```python
from build123d import *

# Parameters (mm, degrees)
SKETCH_1_W                = 73.9
SKETCH_1_H                = 56.9
EXTRUDE_1_DEPTH           = 4
HOLE_WIZARD_1_D           = 3
HOLE_WIZARD_1_CBORE_D     = 6
HOLE_WIZARD_1_CBORE_DEPTH = 2.2
SKETCH_4_W                = 7
SKETCH_4_H                = 25.95
SKETCH_4_W_2              = 33.45
SKETCH_4_H_2              = 7
SKETCH_4_H_3              = 23.95
EXTRUDE_2_DEPTH           = 2
HOLE_WIZARD_2_D           = 3.2
CHAMFER_1_SIZE            = 1
CHAMFER_1_SIZE_2          = 2
CHAMFER_2_SIZE            = 2
CHAMFER_2_SIZE_2          = 1
CHAMFER_3_SIZE            = 2
CHAMFER_3_SIZE_2          = 1
SKETCH_7_W                = 2
SKETCH_7_H                = 1
SKETCH_7_W_2              = 1
SKETCH_7_H_2              = 2
EXTRUDE_3_DEPTH           = 2
FILLET_3_R                = 1
FILLET_4_R                = 1


with BuildPart() as part:
    # 草图1 → 凸台-拉伸1 (new body)
    with BuildSketch(Plane.XY):
        Rectangle(SKETCH_1_W, SKETCH_1_H)
    extrude(amount=EXTRUDE_1_DEPTH)

    # 孔1 (through all)
    with Locations(Plane(origin=(-10, 9.25, 4), x_dir=(1, 0, 0), z_dir=(0, 0, 1))):
        with Locations((0, 0), (20, 0), (20, -18.5), (0, -18.5)):
            CounterBoreHole(HOLE_WIZARD_1_D / 2, HOLE_WIZARD_1_CBORE_D / 2, HOLE_WIZARD_1_CBORE_DEPTH)

    # 草图4 → 凸台-拉伸2 (add)
    with BuildSketch(Plane(origin=(0, 0, 0), x_dir=(-1, 0, 0), z_dir=(0, 0, -1))):
        with BuildLine():
            Line((3.5, 28.45), (3.5, 35.5))
            ThreePointArc((3.5, 35.5), (0, 39), (-3.5, 35.5))
            Line((-3.5, 35.5), (-3.5, 28.45))
            Line((-3.5, 28.45), (3.5, 28.45))
        make_face()
        with Locations((0, 15.475)):
            Rectangle(SKETCH_4_W, SKETCH_4_H)
        with Locations((20.225, -1)):
            Rectangle(SKETCH_4_W_2, SKETCH_4_H_2)
        with BuildLine():
            Line((43, 2.5), (36.95, 2.5))
            Line((36.95, 2.5), (36.95, -4.5))
            Line((36.95, -4.5), (43, -4.5))
            ThreePointArc((43, -4.5), (46.5, -1), (43, 2.5))
        make_face()
        with Locations((0, -1)):
            Rectangle(SKETCH_4_W, SKETCH_4_H_2)
        with Locations((-20.225, -1)):
            Rectangle(SKETCH_4_W_2, SKETCH_4_H_2)
        with Locations((0, -16.475)):
            Rectangle(SKETCH_4_W, SKETCH_4_H_3)
        with BuildLine():
            Line((-36.95, -4.5), (-36.95, 2.5))
            Line((-36.95, 2.5), (-43, 2.5))
            ThreePointArc((-43, 2.5), (-46.5, -1), (-43, -4.5))
            Line((-43, -4.5), (-36.95, -4.5))
        make_face()
        with BuildLine():
            Line((3.5, -35.5), (3.5, -28.45))
            Line((3.5, -28.45), (-3.5, -28.45))
            Line((-3.5, -28.45), (-3.5, -35.5))
            ThreePointArc((-3.5, -35.5), (0, -39), (3.5, -35.5))
        make_face()
    extrude(amount=EXTRUDE_2_DEPTH)

    # 孔2 (through all)
    with Locations(Plane(origin=(43, -1, -2), x_dir=(-1, 0, 0), z_dir=(0, 0, -1))):
        with Locations((0, 0), (43, 36.5), (86, 0), (43, -34.5)):
            Hole(HOLE_WIZARD_2_D / 2)

    # 倒角1
    # the kernel refuses this chamfer: 2, 1 mm, written as the material it adds along each edge
    with BuildSketch(Plane(origin=(-3.5, -2.679657748, 0), x_dir=(-0.9976223042390326, 0, 0.06891834360170879), z_dir=(0, 1, 0))) as chamfer_1_piece_1:
        Polygon((CHAMFER_1_SIZE * 0.997622304239, -CHAMFER_1_SIZE * 0.0689183436017), (-CHAMFER_1_SIZE_2 * 0.0689183436017, -CHAMFER_1_SIZE_2 * 0.997622304239), (0, 0), align=None)
    extrude(amount=31.129657748)
    with BuildSketch(Plane(origin=(-36.95, 2.5, 0), x_dir=(0, 0.9976223042390326, 0.06891834360170879), z_dir=(1, 0, 0))) as chamfer_1_piece_2:
        Polygon((CHAMFER_1_SIZE * 0.997622304239, -CHAMFER_1_SIZE * 0.0689183436017), (-CHAMFER_1_SIZE_2 * 0.0689183436017, -CHAMFER_1_SIZE_2 * 0.997622304239), (0, 0), align=None)
    extrude(amount=38.629657748)

    # 倒角2
    # the kernel refuses this chamfer: 2, 1 mm, written as the material it adds along each edge
    with BuildSketch(Plane(origin=(-3.5, 0.679657748, 0), x_dir=(0.017268075123668084, 0, -0.9998508956747119), z_dir=(0, -1, 0))) as chamfer_2_piece_1:
        Polygon((CHAMFER_2_SIZE * 0.999850895675, -CHAMFER_2_SIZE * 0.0172680751237), (-CHAMFER_2_SIZE_2 * 0.0172680751237, -CHAMFER_2_SIZE_2 * 0.999850895675), (0, 0), align=None)
    extrude(amount=29.129657748)
    with BuildSketch(Plane(origin=(-36.95, -4.5, 0), x_dir=(0, 0.017268075123667872, -0.9998508956747119), z_dir=(1, 0, 0))) as chamfer_2_piece_2:
        Polygon((CHAMFER_2_SIZE * 0.999850895675, -CHAMFER_2_SIZE * 0.0172680751237), (-CHAMFER_2_SIZE_2 * 0.0172680751237, -CHAMFER_2_SIZE_2 * 0.999850895675), (0, 0), align=None)
    extrude(amount=38.629657748)

    # 倒角3
    # the kernel refuses this chamfer: 2, 1 mm, written as the material it adds along each edge
    with BuildSketch(Plane(origin=(3.5, -28.45, 0), x_dir=(-0.0172680751236683, 0, -0.9998508956747119), z_dir=(0, 1, 0))) as chamfer_3_piece_1:
        Polygon((CHAMFER_3_SIZE * 0.999850895675, -CHAMFER_3_SIZE * 0.0172680751237), (-CHAMFER_3_SIZE_2 * 0.0172680751237, -CHAMFER_3_SIZE_2 * 0.999850895675), (0, 0), align=None)
    extrude(amount=29.129657748)
    with BuildSketch(Plane(origin=(-1.679657748, -4.5, 0), x_dir=(0, 0.0172680751236683, -0.9998508956747119), z_dir=(1, 0, 0)), Plane(origin=(36.95, 2.5, 0), x_dir=(0, -0.017268075123667872, -0.9998508956747119), z_dir=(-1, 0, 0))) as chamfer_3_piece_2:
        Polygon((CHAMFER_3_SIZE * 0.999850895675, -CHAMFER_3_SIZE * 0.0172680751237), (-CHAMFER_3_SIZE_2 * 0.0172680751237, -CHAMFER_3_SIZE_2 * 0.999850895675), (0, 0), align=None)
    extrude(amount=38.629657748)
    with BuildSketch(Plane(origin=(3.5, -2.679657748, 0), x_dir=(-0.017268075123668084, 0, -0.9998508956747119), z_dir=(0, 1, 0))) as chamfer_3_piece_3:
        Polygon((CHAMFER_3_SIZE * 0.999850895675, -CHAMFER_3_SIZE * 0.0172680751237), (-CHAMFER_3_SIZE_2 * 0.0172680751237, -CHAMFER_3_SIZE_2 * 0.999850895675), (0, 0), align=None)
    extrude(amount=31.129657748)

    # 草图7 → 凸台-拉伸3 (add)
    # profile 1 of 6: a face of its own
    with BuildSketch(Plane(origin=(0, 0, 0), x_dir=(-1, 0, 0), z_dir=(0, 0, -1))):
        with BuildLine():
            Line((-36.95, 4.5), (-43, 4.5))
            ThreePointArc((-43, 4.5), (-48.5, -1), (-43, -6.5))
            Line((-43, -6.5), (-34.95, -6.5))
            Line((-34.95, -6.5), (-34.95, 3.5))
            Line((-34.95, 3.5), (-36.95, 3.5))
            Line((-36.95, 3.5), (-36.95, 4.5))
        make_face()
        with BuildLine():
            Line((-43, 2.5), (-36.95, 2.5))
            Line((-36.95, 2.5), (-36.95, -4.5))
            Line((-36.95, -4.5), (-43, -4.5))
            ThreePointArc((-43, -4.5), (-46.5, -1), (-43, 2.5))
        make_face(mode=Mode.SUBTRACT)
    # profile 2 of 6: a face of its own
    with BuildSketch(Plane(origin=(0, 0, 0), x_dir=(-1, 0, 0), z_dir=(0, 0, -1))):
        with Locations((-35.95, 4)):
            Rectangle(SKETCH_7_W, SKETCH_7_H)
    # profile 3 of 6: a face of its own
    with BuildSketch(Plane(origin=(0, 0, 0), x_dir=(-1, 0, 0), z_dir=(0, 0, -1))):
        with BuildLine():
            Line((-5.5, -35.5), (-5.5, -26.45))
            Line((-5.5, -26.45), (5.5, -26.45))
            Line((5.5, -26.45), (5.5, -35.5))
            ThreePointArc((5.5, -35.5), (0, -41), (-5.5, -35.5))
        make_face()
        with BuildLine():
            ThreePointArc((-3.5, -35.5), (0, -39), (3.5, -35.5))
            Line((3.5, -35.5), (3.5, -28.45))
            Line((3.5, -28.45), (-3.5, -28.45))
            Line((-3.5, -28.45), (-3.5, -35.5))
        make_face(mode=Mode.SUBTRACT)
    # profile 4 of 6: a face of its own
    with BuildSketch(Plane(origin=(0, 0, 0), x_dir=(-1, 0, 0), z_dir=(0, 0, -1))):
        with BuildLine():
            Line((43, -6.5), (34.95, -6.5))
            Line((34.95, -6.5), (34.95, 4.5))
            Line((34.95, 4.5), (43, 4.5))
            ThreePointArc((43, 4.5), (48.5, -1), (43, -6.5))
        make_face()
        with BuildLine():
            ThreePointArc((43, -4.5), (46.5, -1), (43, 2.5))
            Line((43, 2.5), (36.95, 2.5))
            Line((36.95, 2.5), (36.95, -4.5))
            Line((36.95, -4.5), (43, -4.5))
        make_face(mode=Mode.SUBTRACT)
    # profile 5 of 6: a face of its own
    with BuildSketch(Plane(origin=(0, 0, 0), x_dir=(-1, 0, 0), z_dir=(0, 0, -1))):
        with BuildLine():
            Line((-5.5, 35.5), (-5.5, 28.45))
            Line((-5.5, 28.45), (-4.5, 28.45))
            Line((-4.5, 28.45), (-4.5, 26.45))
            Line((-4.5, 26.45), (5.5, 26.45))
            Line((5.5, 26.45), (5.5, 35.5))
            ThreePointArc((5.5, 35.5), (0, 41), (-5.5, 35.5))
        make_face()
        with BuildLine():
            Line((3.5, 35.5), (3.5, 28.45))
            Line((3.5, 28.45), (-3.5, 28.45))
            Line((-3.5, 28.45), (-3.5, 35.5))
            ThreePointArc((-3.5, 35.5), (0, 39), (3.5, 35.5))
        make_face(mode=Mode.SUBTRACT)
    # profile 6 of 6: a face of its own
    with BuildSketch(Plane(origin=(0, 0, 0), x_dir=(-1, 0, 0), z_dir=(0, 0, -1))):
        with Locations((-5, 27.45)):
            Rectangle(SKETCH_7_W_2, SKETCH_7_H_2)
    extrude(amount=EXTRUDE_3_DEPTH)

    # 圆角3
    fillet_3_edges = [part.edges().sort_by_distance(p)[0] for p in [
        (-34.95, -6.5, -1),
        (-34.95, 4.5, -1),
        (5.5, -26.45, -1),
        (-5.5, -26.45, -1),
        (-5.5, 26.45, -1),
        (5.5, 26.45, -1),
        (34.95, 4.5, -1),
        (34.95, -6.5, -1),
    ]]
    fillet(fillet_3_edges, radius=FILLET_3_R)

    # 圆角4
    fillet_4_edges = [part.edges().sort_by_distance(p)[0] for p in [
        (36.95, -28.45, 2),
        (-36.95, -28.45, 2),
        (-36.95, 28.45, 2),
        (36.95, 28.45, 2),
    ]]
    fillet(fillet_4_edges, radius=FILLET_4_R)


solid = part.part
```
Check sheet for the modelled part. Datum: model origin and axes. Units: mm. A direction names the side the tool comes from. Coordinates: 2 decimals unless noted, no trailing zeros. Order: outer loops, then holes, each group sorted by start corner. A loop starts at its lowest first (then second) coordinate and runs counter-clockwise, first axis right, second up. Notation, with made-up numbers: (64, 47) -> (104, 47) arc R8 cw to (104, 51) -> close; hole circle Ø6 at (26.5, 41). An arc over 180 degrees is marked (long way). Write item = value, one per line. Start each with the question number.
1) Access from +Z, -Z, +X, -X, +Y, -Y to the whole of each face (thin tool, end or side, straight path). Record for faces 1 (the flat face through (-1, 0, 4)), 2 (the flat face through (-9, -11, 1.8)), 3 (the flat face through (41.5, -2.1, 0)).
2) Cross-section at B-B (z = 3). Enter the section's corners in (x, y), then the cut area to 3 significant figures.
3) Go/stop test with flat-tipped pins: P1, Ø1.1, axis at y = -5, z = -1, coming from the -X side; P2, Ø5, axis at x = 0, y = 35.5, coming from the +Z side; P3, Ø1.5, axis at y = 7, z = 0, coming from the -X side. Record where each tip stops, or that it passes through.
4) Cross-section at D-D (x = -19.5). Enter the section's corners in (y, z).
5) Material ranges on L1, parallel to Y at x = 10, z = 0.95; L2, parallel to Y at x = -43, z = -1.5; L3, parallel to Y at x = -5, z = -1, recorded low to high.
6) Cross-section at C-C (x = 0). Enter the section's corners in (y, z).
7) Mould release check, pull along Y, two halves, no side actions. Record for faces 4 (the flat face through (-5.5, -31, -1)), 5 (the cylindrical face through (-48.5, -0.9, -1)), 6 (the cylindrical face through (41.82, 0.08, -0.99)): +Y half, -Y half, draft (parallel to the pull), parting line (faces both ways), or undercut.
8) Cross-section at A-A (y = -1). Enter the section's corners in (x, z), then the cut area to 3 significant figures.
Ans:
q1.face_1 = +Z, +X, -X, +Y, -Y
q1.face_2 = +Z
q1.face_3 = +Z, +X, +Y, -Y
q2.outline = (-36.95, -27.45) arc R1 ccw to (-35.95, -28.45) -> (35.95, -28.45) arc R1 ccw to (36.95, -27.45) -> (36.95, 27.45) arc R1 ccw to (35.95, 28.45) -> (-35.95, 28.45) arc R1 ccw to (-36.95, 27.45) -> close; hole circle Ø6 at (-10, -9.25); hole circle Ø6 at (-10, 9.25); hole circle Ø6 at (10, -9.25); hole circle Ø6 at (10, 9.25)
q2.area = 4,090 mm²
q3.P1 = -47.28
q3.P2 = 0
q3.P3 = -36.95
q4.outline = (-28.45, 0) -> (-5.5, 0) -> (-4.5, -2) -> (2.5, -2) -> (3.5, 0) -> (28.45, 0) -> (28.45, 4) -> (-28.45, 4) -> close
q5.L1 = -28.45 to -10.75, -7.75 to 7.75, 10.75 to 28.45
q5.L2 = -6.5 to -2.6, 0.6 to 4.5
q5.L3 = -37.79 to -26.58, -5 to 3, 26.58 to 37.79
q6.outline = (-41, -2) -> (-37.1, -2) -> (-37.1, 0) -> (-41, 0) -> close; (-33.9, -2) -> (33.9, -2) -> (33.9, 0) -> (28.45, 0) -> (28.45, 4) -> (-28.45, 4) -> (-28.45, 0) -> (-33.9, 0) -> close; (37.1, -2) -> (41, -2) -> (41, 0) -> (37.1, 0) -> close
q7.face_4 = draft
q7.face_5 = parting line
q7.face_6 = undercut
q8.outline = (-48.5, -2) -> (-44.6, -2) -> (-44.6, 0) -> (-48.5, 0) -> close; (-41.4, -2) -> (41.4, -2) -> (41.4, 0) -> (36.95, 0) -> (36.95, 4) -> (-36.95, 4) -> (-36.95, 0) -> (-41.4, 0) -> close; (44.6, -2) -> (48.5, -2) -> (48.5, 0) -> (44.6, 0) -> close
q8.area = 477 mm²
